Here's how the part is built. I have some questions about the finished solid (model axes, mm). A direction names the side the tool comes from. Coordinates: 2 decimals unless noted, no trailing zeros. Order: outer loops, then holes, each group sorted by start corner. A loop starts at its lowest first (then second) coordinate and runs counter-clockwise, first axis right, second up. Notation, with made-up numbers: (51.25, 21.25) - (76.25, 21.25) arc R25 ccw to (76.25, 36.25) - close; hole circle Ø7 at (-9.5, 16.5). An arc over 180 degrees is marked (long way). Use CSV: the item, a comma, the result in double quotes. Start each with the question number.
from build123d import *

# Parameters (mm, degrees)
BOSS_EXTRUDE1_DEPTH    = 35
SKETCH4_W              = 1200
SKETCH4_H              = 805.2
BOSS_EXTRUDE2_DEPTH    = 6.35
CHAMFER1_SIZE          = 10
F_20_0MM_DOWEL_HOLE1_D = 21


with BuildPart() as part:
    # Sketch3 → Boss-Extrude1 (new body)
    with BuildSketch(Plane(origin=(0, 0, 0), x_dir=(1, 0, 0), z_dir=(0, 1, 0))):
        with BuildLine():
            Line((0, 541), (0, 521))
            ThreePointArc((0, 521), (-260.5, 451.199235372), (-451.199235372, 260.5))
            Line((-451.199235372, 260.5), (-468.519743447, 270.5))
            ThreePointArc((-468.519743447, 270.5), (-270.5, 468.519743447), (0, 541))
        make_face()
    extrude(amount=BOSS_EXTRUDE1_DEPTH)

    # Sketch4 → Boss-Extrude2 (add)
    with BuildSketch(Plane(origin=(0, 0, 0), x_dir=(1, 0, 0), z_dir=(0, 1, 0))):
        with Locations((-154.139235372, 138.4)):
            Rectangle(SKETCH4_W, SKETCH4_H)
    extrude(amount=-BOSS_EXTRUDE2_DEPTH)

    # Chamfer1
    # the kernel refuses this chamfer: 10 mm, written as the material it takes off along each edge
    with BuildSketch(Plane(origin=(0, 0, -521), x_dir=(-0.999953038196086, 0, 0.009691305506332204), z_dir=(0, 1, 0))) as chamfer1_piece_1:
        with BuildLine():
            Line((10.098340338, 0), (-CHAMFER1_SIZE * 0.00969130550633, -CHAMFER1_SIZE * 0.999953038196))
            Line((-CHAMFER1_SIZE * 0.00969130550633, -CHAMFER1_SIZE * 0.999953038196), (0, 0))
            ThreePointArc((0, 0), (5.192000536, -0.024447522), (10.098340338, 0))
        make_face()
    extrude(amount=60.969219121, mode=Mode.SUBTRACT)

    # Ø20.0mm Dowel Hole1 (through all)
    with Locations(Plane(origin=(0, 0, 0), x_dir=(1, 0, 0), z_dir=(0, 1, 0))):
        with Locations((0, 0)):
            Hole(F_20_0MM_DOWEL_HOLE1_D / 2)


solid = part.part
Item 1: Suppose I cut it at C-C on z = -485.5. Write out the boundary of the cut face in (x, y).
Item 2: Please list where these lines run through material, in increasing order: line 1 along Z through (x, y) = (0, -2.25); line 2 along Y through (x, z) = (-314.5, 184.5); line 3 along Z through (x, y) = (-394, 10). Write a range as from..to.
Item 3: Suppose I cut it at D-D on z = -165. Write out the boundary of the cut face in (x, y).
Item 4: Suppose I cut it at A-A on y = 24. Write out the boundary of the cut face in (x, z).
Item 5: For faces 1 (the cylindrical face through (-261.626, 17.255, -450.547)), 2 (the flat face through (-163, -6.35, -144)), 3 (the cylindrical face through (-273.927, 17.255, -466.524)), which set-ups out of +Z, -Z, +X, -X, +Y, -Y let a thin tool reach every point of the face, with its end or its side?
Item 6: Suppose I cut it at B-B on x = -254. Write out the boundary of the cut face in (y, z).
Item 7: For pin 1 Ø3 at (y, z) = (7, -342) entering from +X; pin 2 Ø2 at (x, z) = (303.5, -221.5) entering from +Y; pin 3 Ø3 at (y, z) = (10, -538.5) entering from +X, each with a flat end and sliding along its axis, tell me the tip position at first contact or that it passes through.
Here are the results:
1,outline,"(-754.14, -6.35) - (445.86, -6.35) - (445.86, 0) - (-189.03, 0) - (-189.03, 35) - (-238.69, 35) - (-238.69, 0) - (-754.14, 0) - close"
2,line 1,"-541..-10.5, 10.5..264.2"
2,line 2,"-6.35..0"
2,line 3,"-370.74..-340.89"
3,outline,"(-754.14, -6.35) - (445.86, -6.35) - (445.86, 0) - (-754.14, 0) - close"
4,outline,"(-468.52, -270.5) arc R541 ccw to (0, -541) - (0, -531) - (-10.1, -520.9) arc R521 cw to (-451.2, -260.5) - close"
5,face 1,"+Z, +X, +Y"
5,face 2,"+Z, -Z, +X, -X, -Y"
5,face 3,"-Z, -X, +Y"
6,outline,"(-6.35, -541) - (0, -541) - (0, -477.67) - (35, -477.67) - (35, -454.89) - (0, -454.89) - (0, 264.2) - (-6.35, 264.2) - close"
7,pin 1,"x = -391.73"
7,pin 2,"y = 0"
7,pin 3,"x = 0"
